Source: CAD feature listing. Evaluate the final solid. Frame: model axes, mm. Round coordinates to 2 decimals unless told otherwise and drop trailing zeros. Order: outer loops, then holes, each group sorted by start corner. A loop starts at its lowest first (then second) coordinate and runs counter-clockwise, first axis right, second up. Notation, with made-up numbers: (-35, 60) - (16, 60) arc R28 cw to (16, 88) - close; hole circle Ø9 at (84.5, -14.75). An arc over 180 degrees is marked (long way). Return JSON: item names as keys, results as strings. Group by question number.
1) Ray query, line 1 (Y direction, x = -3, z = 3.25); line 2 (Y direction, x = 22.5, z = 3.8); line 3 (X direction, y = 0.5, z = 2.05). Return the intervals inside material, ascending. Write a range as from..to.
2) Section A-A, the plane y = -17.5. Return loops of the section in (x, z).
3) Contact query for flat-ended pins moving along their axis: P1, Ø5.5, axis at x = -19.5, y = -39, coming from the -Z side; P2, Ø1.5, axis at x = -2.5, z = 2, coming from the +Y side. Output: stop coordinate, or through.
4) Section B-B, the plane z = 1.6. Give the number of separate pieces and of enclosed holes in the cut face, plus the area to 3 significant figures.
5) Section C-C, the plane y = 40.5. Return loops of the section in (x, z), plus the area to 3 significant figures.
6) Section D-D, the plane y = -39. Return loops of the section in (x, z), plus the area to 3 significant figures.
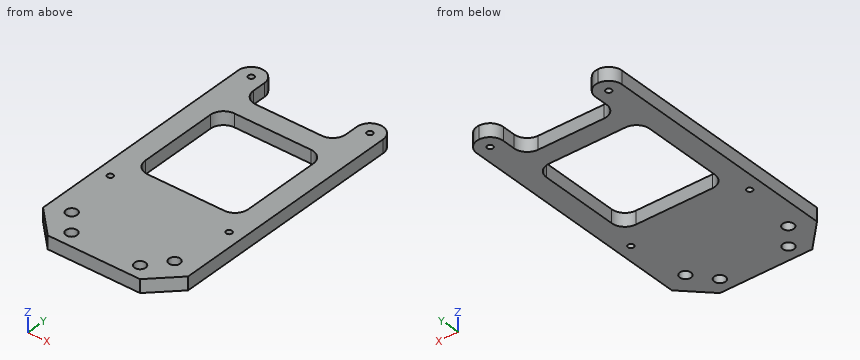
```python
from build123d import *

# Parameters (mm, degrees)
SKETCH_1_W          = 55
SKETCH_1_H          = 105
SKETCH_1_R          = 1.1
EXTRUDE_1_DEPTH     = 5
CHAMFER_1_SIZE      = 10
SKETCH_4_R          = 2.1
CUT_EXTRUDE_1_DEPTH = 10
SKETCH_5_W          = 35
SKETCH_5_H          = 15
CUT_EXTRUDE_2_DEPTH = 10
SKETCH_6_W          = 39
SKETCH_6_H          = 40
CUT_EXTRUDE_3_DEPTH = 10
FILLET_3_R          = 5
FILLET_4_R          = 5


with BuildPart() as part:
    # 草图1 → 凸台-拉伸1 (new body)
    with BuildSketch(Plane.XY):
        Rectangle(SKETCH_1_W, SKETCH_1_H)
        with Locations((-22.5, 47.5)):
            Circle(SKETCH_1_R, mode=Mode.SUBTRACT)
        with Locations(Location((22.5, 47.5, 0), (0, 0, 180))):
            Circle(SKETCH_1_R, mode=Mode.SUBTRACT)
        with Locations((-22.5, -17.5)):
            Circle(SKETCH_1_R, mode=Mode.SUBTRACT)
        with Locations(Location((22.5, -17.5, 0), (0, 0, 180))):
            Circle(SKETCH_1_R, mode=Mode.SUBTRACT)
    extrude(amount=EXTRUDE_1_DEPTH)

    # 倒角1
    chamfer_1_edges = [part.edges().sort_by_distance(p)[0] for p in [
        (27.5, -52.5, 2.5),
        (-27.5, -52.5, 2.5),
    ]]
    chamfer(chamfer_1_edges, length=CHAMFER_1_SIZE)

    # 草图4 → 切除-拉伸1 (cut)
    with BuildSketch(Plane(origin=(0, 0, 0), x_dir=(-1, 0, 0), z_dir=(0, 0, -1))):
        with Locations((-13, -47)):
            Circle(SKETCH_4_R)
        with Locations((-19.5, -39)):
            Circle(SKETCH_4_R)
        with Locations(Location((19.5, -39, 0), (0, 0, 180))):
            Circle(SKETCH_4_R)
        with Locations(Location((13, -47, 0), (0, 0, 180))):
            Circle(SKETCH_4_R)
    extrude(amount=-CUT_EXTRUDE_1_DEPTH, mode=Mode.SUBTRACT)

    # 草图5 → 切除-拉伸2 (cut)
    with BuildSketch(Plane.XY.offset(5)):
        with Locations((0, 45)):
            Rectangle(SKETCH_5_W, SKETCH_5_H)
    extrude(amount=-CUT_EXTRUDE_2_DEPTH, mode=Mode.SUBTRACT)

    # 草图6 → 切除-拉伸3 (cut)
    with BuildSketch(Plane.XY.offset(5)):
        with Locations((0, 10)):
            Rectangle(SKETCH_6_W, SKETCH_6_H)
    extrude(amount=-CUT_EXTRUDE_3_DEPTH, mode=Mode.SUBTRACT)

    # 圆角3
    fillet_3_edges = [part.edges().sort_by_distance(p)[0] for p in [
        (19.5, 30, 2.5),
        (19.5, -10, 2.5),
        (-19.5, -10, 2.5),
        (-19.5, 30, 2.5),
    ]]
    fillet(fillet_3_edges, radius=FILLET_3_R)

    # 圆角4
    fillet_4_edges = [part.edges().sort_by_distance(p)[0] for p in [
        (17.5, 52.5, 2.5),
        (27.5, 52.5, 2.5),
        (-27.5, 52.5, 2.5),
        (-17.5, 52.5, 2.5),
        (17.5, 37.5, 2.5),
        (-17.5, 37.5, 2.5),
    ]]
    fillet(fillet_4_edges, radius=FILLET_4_R - 0.0001)  # a hair under: the kernel refuses the full size


solid = part.part
```
Geometry check:
{
 "1": {"line 1": "-52.5..-10, 30..37.5", "line 2": "-47.5..-18.6, -16.4..46.4, 48.6..52.5", "line 3": "-27.5..-19.5, 19.5..27.5"},
 "2": {"outline": "(-27.5, 0) - (-23.6, 0) - (-23.6, 5) - (-27.5, 5) - close; (-21.4, 0) - (21.4, 0) - (21.4, 5) - (-21.4, 5) - close; (23.6, 0) - (27.5, 0) - (27.5, 5) - (23.6, 5) - close"},
 "3": {"P1": "z = 0", "P2": "y = 37.5"},
 "4": {"separate pieces": "1", "enclosed holes": "9", "area": "3,530 mm2"},
 "5": {"outline": "(-27.5, 0) - (-17.08, 0) - (-17.08, 5) - (-27.5, 5) - close; (17.08, 0) - (27.5, 0) - (27.5, 5) - (17.08, 5) - close", "area": "104 mm2"},
 "6": {"outline": "(-27.5, 0) - (-21.6, 0) - (-21.6, 5) - (-27.5, 5) - close; (-17.4, 0) - (17.4, 0) - (17.4, 5) - (-17.4, 5) - close; (21.6, 0) - (27.5, 0) - (27.5, 5) - (21.6, 5) - close", "area": "233 mm2"}
}
